Work out the finished part from the listing and answer in its coordinate system (mm). A direction names the side the tool comes from. Coordinates: 2 decimals unless noted, no trailing zeros. Order: outer loops, then holes, each group sorted by start corner. A loop starts at its lowest first (then second) coordinate and runs counter-clockwise, first axis right, second up. Notation, with made-up numbers: (1.25, 6.5) - (35.25, 6.5) arc R21 ccw to (35.25, 41.5) - close; hole circle Ø1 at (-24, 33). An arc over 180 degrees is marked (long way). Answer as a JSON object with one key per item and string values. Group by question number.
1) A tool of negligible diameter and unlimited length cuts with its end or side. For faces 4 (the face through (-25.16, 3.06, -7.39)), 5 (the face through (0, 0, 0)), from which of +Z, -Z, +X, -X, +Y, -Y can it reach the whole face along a straight path? Write none if from no direction.
2) Each of these flat-tipped pins is pushed along its axis until it touches: P1, Ø1, axis at x = -25, y = -9, coming from the +Z side; P2, Ø1.5, axis at y = 10, z = 3, coming from the +X side; P3, Ø1.5, axis at x = -41, z = 1.5, coming from the -Y side; P4, Ø5, axis at x = -46, z = -7.5, coming from the -Y side (3 decimals). Where does it stop, or does it pass through?
3) Section D-D (x = -33.5) is taken. Give the vertices of the cut face in (y, z).
4) Section C-C (x = -5) is taken. Give the vertices of the cut face in (y, z), plus the area to 3 significant figures.
5) Section B-B (y = 0) is taken. Give the vertices of the cut face in (x, z).
6) The mould has two halves that part along X. Classify faces 1 (the face through (-52.479, -3.755, -11.923)), 2 (the face through (-2.89, 0.11, 1.34)), 3 (the face through (-55, 0, 0)): released by +X, released by -X, zero draft, split by the parting line, or undercut.
7) Find the intervals of material crossed by line 1 along X through (y, z) = (2.5, 0); line 2 along X through (y, z) = (-1.75, -10); line 3 along Z through (x, y) = (-5, -4), in increasing order.
8) Section A-A (z = 0) is taken. Give the vertices of the cut face in (x, y), plus the area to 3 significant figures.
from build123d import *

# Parameters (mm, degrees)
CHAMFER_1_SIZE      = 1
CHAMFER_2_SIZE      = 1
SKETCH_2_R          = 2.5
CUT_EXTRUDE_1_DEPTH = 40


with BuildPart() as part:
    # 草图1 → 旋转1 (revolve)
    with BuildSketch(Plane.XY, mode=Mode.PRIVATE) as revolve_1_sk:
        Polygon((-55, 0), (-55, 12.5), (-50, 12.5), (-50, 8), (0, 8), (0, 0), align=None)
    revolve(revolve_1_sk.sketch.rotate(Axis((0, 0, 0), (-1, 0, 0)), 90), axis=Axis((0, 0, 0), (-1, 0, 0)))

    # 倒角1
    chamfer_1_edges = [part.edges().sort_by_distance(p)[0] for p in [
        (-50, 0, 12.5),
        (-55, 0, 12.5),
    ]]
    chamfer(chamfer_1_edges, length=CHAMFER_1_SIZE)

    # 倒角2
    chamfer_2_edges = [part.edges().sort_by_distance(p)[0] for p in [
        (0, 0, 8),
    ]]
    chamfer(chamfer_2_edges, length=CHAMFER_2_SIZE)

    # 草图2 → 切除-拉伸1 (cut, symmetric)
    with BuildSketch(Plane(origin=(0, 0, 0), x_dir=(1, 0, 0), z_dir=(0, 1, 0))):
        with Locations(Location((-5, 0, 0), (0, 0, 270))):
            Circle(SKETCH_2_R)
    extrude(amount=CUT_EXTRUDE_1_DEPTH, both=True, mode=Mode.SUBTRACT)


solid = part.part
Report:
{
 "1": {"face 4": "+X", "face 5": "+Z, -Z, +X, +Y, -Y"},
 "2": {"P1": "passes through", "P2": "stops at x = -50", "P3": "stops at y = -7.96", "P4": "stops at y = -6.245"},
 "3": {"outline": "circle Ø16 at (0, 0)"},
 "4": {"outline": "(-7.6, -2.5) arc R8 ccw to (7.6, -2.5) - close; (-7.6, 2.5) - (7.6, 2.5) arc R8 ccw to start", "area": "122 mm²"},
 "5": {"outline": "(-55, -11.5) - (-54, -12.5) - (-51, -12.5) - (-50, -11.5) - (-50, -8) - (-1, -8) - (0, -7) - (0, 7) - (-1, 8) - (-50, 8) - (-50, 11.5) - (-51, 12.5) - (-54, 12.5) - (-55, 11.5) - close; hole circle Ø5 at (-5, 0)"},
 "6": {"face 1": "zero draft", "face 2": "undercut", "face 3": "released by -X"},
 "7": {"line 1": "x = -55 to -7.5, -2.5 to 0", "line 2": "x = -55 to -50", "line 3": "z = -6.93 to -2.5, 2.5 to 6.93"},
 "8": {"outline": "(-55, -11.5) - (-54, -12.5) - (-51, -12.5) - (-50, -11.5) - (-50, -8) - (-7.5, -8) - (-7.5, 8) - (-50, 8) - (-50, 11.5) - (-51, 12.5) - (-54, 12.5) - (-55, 11.5) - close; (-2.5, -8) - (-1, -8) - (0, -7) - (0, 7) - (-1, 8) - (-2.5, 8) - close", "area": "842 mm²"}
}
